CAD build for the part. Positions are in the model's coordinates, mm. A direction names the side the tool comes from. Round coordinates to 2 decimals unless told otherwise and drop trailing zeros. Write each loop counter-clockwise with the first axis right and the second up, starting at its lowest first coordinate (ties: lowest second). Pieces come first, ordered by that corner, then holes. Notation, with made-up numbers: M 74,34.25 L 107,34.25 A13 ccw 107,43.25 Z; hole C 24.25,62.25 d2. An arc over 180 degrees is marked long. Write each question's results on one line, items separated by ' | '. Start each with the question number.
```python
from build123d import *

# Parameters (mm, degrees)
F0_W     = 6.884935
F0_H     = 17.032009
F1_DEPTH = 25.4


with BuildPart() as f1:
    # F0 (on Front) → F1 (new body)
    with BuildSketch(Plane.XZ):
        with BuildLine():
            Line((0, -6.35), (0, 0))
            Line((0, 0), (0, 6.35))
            Line((0, 6.35), (0, 15.24))
            ThreePointArc((0, 15.24), (-4.463693, 4.463693), (-15.24, 0))
            Line((-15.24, 0), (-138.150647, 0))
            ThreePointArc((-138.150647, 0), (-149.841652, -11.691004), (-138.150647, -23.382009))
            Line((-138.150647, -23.382009), (-100.798674, -23.382009))
            Line((-100.798674, -23.382009), (0, -23.382009))
            Line((0, -23.382009), (165.1, -23.382009))
            ThreePointArc((165.1, -23.382009), (179.966004, -8.516004), (165.1, 6.35))
            Line((165.1, 6.35), (12.470275, 6.35))
            Line((12.470275, 6.35), (11.642048, 6.35))
            Line((11.642048, 6.35), (11.642048, 5.319719))
            Line((11.642048, 5.319719), (11.642048, 1.030281))
            Line((11.642048, 1.030281), (11.642048, 0))
            Line((11.642048, 0), (12.470275, 0))
            Line((12.470275, 0), (20.300698, 0))
            Line((20.300698, 0), (20.300698, -17.032009))
            Line((20.300698, -17.032009), (0, -17.032009))
            Line((0, -17.032009), (0, -6.35))
        make_face()
        with BuildLine():
            ThreePointArc((-15.24, -6.35), (-6.217977, -9.307464), (-0.697568, -17.032009))
            Line((-0.697568, -17.032009), (-100.798674, -17.032009))
            Line((-100.798674, -17.032009), (-138.150647, -17.032009))
            ThreePointArc((-138.150647, -17.032009), (-143.491652, -11.691004), (-138.150647, -6.35))
            Line((-138.150647, -6.35), (-15.24, -6.35))
        make_face(mode=Mode.SUBTRACT)
        with Locations((28.442165, -8.516004)):
            Rectangle(F0_W, F0_H, mode=Mode.SUBTRACT)
        with BuildLine():
            ThreePointArc((165.1, 0), (173.616004, -8.516004), (165.1, -17.032009))
            Line((165.1, -17.032009), (36.583633, -17.032009))
            Line((36.583633, -17.032009), (36.583633, 0))
            Line((36.583633, 0), (165.1, 0))
        make_face(mode=Mode.SUBTRACT)
        with BuildLine():
            ThreePointArc((8.959904, 0), (10.396513, 0.266429), (11.642048, 1.030281))
            Line((11.642048, 1.030281), (11.642048, 5.319719))
            ThreePointArc((11.642048, 5.319719), (10.396513, 6.083571), (8.959904, 6.35))
            Line((8.959904, 6.35), (4.699, 6.35))
            Line((4.699, 6.35), (4.699, 0))
            Line((4.699, 0), (8.959904, 0))
        make_face()
    extrude(amount=F1_DEPTH)


solid = f1.part
```
1) Pull direction Z, two halves, no side cores. Call faces 1 (the face through (102, -13, -17.032)), 2 (the face through (4.699, -13, 3)), 3 (the face through (-149.84, -12.52, -11.43)): pulls with the +Z half, pulls with the -Z half, needs draft (parallel to the pull), parting line crosses it, or undercut.
2) Saw through at C-C, the plane z = -3.5. Write the cut outline in (x, y), plus the area to 3 significant figures.
3) Wall check: line 1 along X through (y, z) = (-8.25, -11); line 2 along X through (y, z) = (-21, -10.5); line 3 along Z through (x, y) = (42, -15). Give the ranges that are in metal, low to high. Write a range as from..to.
4) Saw through at D-D, the plane x = -5.5. Write the cut outline in (y, z).
5) Drop flat-ended pins along their axis: pin 1 Ø2 at (x, y) = (28, -12.5) entering from +Z; pin 2 Ø1.5 at (y, z) = (-17, -0.5) entering from -X; pin 3 Ø1 at (x, y) = (-87, -6.5) entering from +Z. Give the stop position or say it passes through.
6) 3-axis set-ups, long thin cutter, end or side, ignore diameter. For faces 4 (the face through (10, -13, -17.032)), 5 (the face through (-76, -13, 0)), 6 (the face through (0, -13, -1)): which of +Z, -Z, +X, -X, +Y, -Y reach the whole face in a straight line?
7) Saw through at B-B, the plane x = 110.5. Write the cut outline in (y, z), plus the area to 3 significant figures.
8) Saw through at A-A, the plane y = -7. State how many separate pieces and enclosed holes the cut face has, plus the area to 3 significant figures.
Filled sheet:
1) face 1: undercut | face 2: needs draft | face 3: parting line crosses it
2) outline: M -146.49,-25.4 L 0,-25.4 L 0,0 L -146.49,0 Z; M 20.3,-25.4 L 25,-25.4 L 25,0 L 20.3,0 Z; M 31.88,-25.4 L 36.58,-25.4 L 36.58,0 L 31.88,0 Z; M 171.98,-25.4 L 179.09,-25.4 L 179.09,0 L 171.98,0 Z | area: 4,140 mm^2
3) line 1: x = -149.82..-143.45, -4.28..0, 20.3..25, 31.88..36.58, 173.25..179.76 | line 2: x = -149.78..-143.36, -4.79..0, 20.3..25, 31.88..36.58, 173.38..179.83 | line 3: z = -23.38..-17.03, 0..6.35
4) outline: M -25.4,-23.38 L 0,-23.38 L 0,-17.03 L -25.4,-17.03 Z; M -25.4,-9.87 L 0,-9.87 L 0,3.52 L -25.4,3.52 Z
5) pin 1: stops at z = 6.35 | pin 2: stops at x = -143.41 | pin 3: stops at z = 0
6) face 4: +Y, -Y | face 5: +Z, -X, +Y, -Y | face 6: +Z, +Y, -Y
7) outline: M -25.4,-23.38 L 0,-23.38 L 0,-17.03 L -25.4,-17.03 Z; M -25.4,0 L 0,0 L 0,6.35 L -25.4,6.35 Z | area: 323 mm^2
8) separate pieces: 1 | enclosed holes: 3 | area: 4,480 mm^2
